The listing builds one solid part. Answer for the finished solid, in the listing's coordinates (mm). A direction names the side the tool comes from. Round coordinates to 2 decimals unless told otherwise and drop trailing zeros. Order: outer loops, then holes, each group sorted by start corner. A loop starts at its lowest first (then second) coordinate and runs counter-clockwise, first axis right, second up. Notation, with made-up numbers: (-2, -34) - (36, -34) arc R27 ccw to (36, 0) - close; hole circle Ø8 at (71.25, -36). An arc over 180 degrees is marked (long way). One line per item, written item: value. Start each with the question number.
1. Section B-B, the plane x = -21 is taken. Give the vertices of the cut face in (y, z), then the cut area to 3 significant figures.
2. Straight lines are drawn through the part: line 1 (Y direction, x = 0, z = 3.5); line 2 (Y direction, x = -46.5, z = 2.4); line 3 (Y direction, x = -7, z = 5.5). For each, find the intervals that lie inside material, in ascending order.
3. For a pull along X with two mould halves and no side action, classify faces 3 (the flat face through (-69.85, -92, 3)), 4 (the flat face through (-1, -31, 0)), 5 (the cylindrical face through (58.03, -62.15, 2.96)), 6 (the cylindrical face through (0.577, 38.096, 2.88)) as released by +X, released by -X, zero draft, split by the parting line, or undercut.
4. Flat-ended cylindrical pins translate along their axes: P1, Ø5.5, axis at x = 0, y = 0, coming from the -Z side; P2, Ø3, axis at y = -91, z = 3.5, coming from the -X side; P3, Ø3, axis at x = -16, z = 4, coming from the +Y side; P4, Ø3, axis at y = -91.5, z = 2, coming from the +X side. Find the tip coordinate at first contact, or state that the pin passes through.
5. Section A-A, the plane y = 0 is taken. Give the vertices of the cut face in (x, z), then the cut area to 3 significant figures.
6. Section C-C, the plane z = 3.95 is taken. Count the separate pieces of the cut face and the enclosed holes in it, then the cut area to 3 significant figures.
7. A tool of negligible diameter and unlimited length cuts with its end or side. For faces 1 (the flat face through (61, -33.6, 2.9)), 2 (the flat face through (-19, -95.25, 3)), from which of +Z, -Z, +X, -X, +Y, -Y can it reach the whole face along a straight path? Write none if from no direction.
8. Section D-D, the plane x = 16.5 is taken. Give the vertices of the cut face in (y, z).
from build123d import *

# Parameters (mm, degrees)
F1_DEPTH = 5.842
F2_R     = 2.9845
F2_R_2   = 4.7625
F3_DEPTH = 25.4
F4_W     = 25.4
F4_H     = 5.842
F5_DEPTH = 25.4


with BuildPart() as f1:
    # F0 (on Top) → F1 (new body)
    with BuildSketch(Plane.XY):
        with BuildLine():
            ThreePointArc((0, -38.1), (26.940768, -26.940768), (38.1, 0))
            ThreePointArc((38.1, 0), (36.969278, 9.21317), (33.644225, 17.879489))
            ThreePointArc((33.644225, 17.879489), (0, 38.1), (-33.644225, 17.879489))
            ThreePointArc((-33.644225, 17.879489), (-32.655922, -19.626532), (0, -38.1))
        make_face()
        with BuildLine():
            ThreePointArc((33.644225, 17.879489), (36.969278, 9.21317), (38.1, 0))
            ThreePointArc((38.1, 0), (26.940768, -26.940768), (0, -38.1))
            ThreePointArc((0, -38.1), (-32.655922, -19.626532), (-33.644225, 17.879489))
            Line((-33.644225, 17.879489), (-87.637326, -83.720511))
            Line((-87.637326, -83.720511), (-101.6, -101.6))
            Line((-101.6, -101.6), (-53.993101, -101.6))
            Line((-53.993101, -101.6), (53.993101, -101.6))
            Line((53.993101, -101.6), (101.6, -101.6))
            Line((101.6, -101.6), (87.637326, -83.720511))
            Line((87.637326, -83.720511), (33.644225, 17.879489))
        make_face()
        Polygon((-13.498275, -63.5), (0, -38.1), (13.498275, -63.5), (22.416117, -80.280898), (-22.416117, -80.280898), align=None, mode=Mode.SUBTRACT)
        Polygon((13.498275, -63.5), (-13.498275, -63.5), (-22.416117, -80.280898), (22.416117, -80.280898), align=None)
    extrude(amount=F1_DEPTH)

    # F2 (on face) → F3 (cut)
    with BuildSketch(Plane.XY.offset(5.842)):
        Circle(F2_R)
        with Locations((53.631348, -60.325)):
            Circle(F2_R_2)
    extrude(amount=-F3_DEPTH, mode=Mode.SUBTRACT)

    # F4 (on face) → F5 (cut)
    with BuildSketch(Plane.XY.offset(5.842)):
        with Locations((-57.15, -92.329)):
            Rectangle(F4_W, F4_H)
        with Locations((-19.05, -92.329)):
            Rectangle(F4_W, F4_H)
    extrude(amount=-F5_DEPTH, mode=Mode.SUBTRACT)


solid = f1.part
Answer list:
1. outline: (-101.6, 0) - (-95.25, 0) - (-95.25, 5.84) - (-101.6, 5.84) - close; (-89.41, 0) - (31.79, 0) - (31.79, 5.84) - (-89.41, 5.84) - close
1. area: 745 mm²
2. line 1: y = -101.6 to -63.5, -38.1 to -2.98, 2.98 to 38.1
2. line 2: y = -101.6 to -95.25, -89.41 to -6.31
2. line 3: y = -101.6 to -95.25, -89.41 to -63.5, -51.27 to 37.45
3. face 3: undercut
3. face 4: zero draft
3. face 5: undercut
3. face 6: split by the parting line
4. P1: passes through
4. P2: stops at x = -94.49
4. P3: stops at y = 35.23
4. P4: stops at x = 94.88
5. outline: (-43.15, 0) - (-2.98, 0) - (-2.98, 5.84) - (-43.15, 5.84) - close; (2.98, 0) - (43.15, 0) - (43.15, 5.84) - (2.98, 5.84) - close
5. area: 469 mm²
6. separate pieces: 1
6. enclosed holes: 5
6. area: 15,900 mm²
7. face 1: +Z, -Z, +X, +Y
7. face 2: +Z, -Z
8. outline: (-101.6, 0) - (34.34, 0) - (34.34, 5.84) - (-101.6, 5.84) - close
